Input: part model. Units: mm. Frame: model coordinates. Face numbers are marked on the shaded views. A direction names the side the tool comes from. Coordinates: 2 decimals unless noted, no trailing zeros. Order: outer loops, then holes, each group sorted by start corner. A loop starts at its lowest first (then second) coordinate and runs counter-clockwise, first axis right, second up. Notation, with made-up numbers: (7, 68.5) -> (40, 68.5) arc R20 cw to (40, 74.5) -> close; hole circle Ø3 at (-0.75, 83.5). An arc over 180 degrees is marked (long way). One line per item, written item: value. Start each with the question number.
from build123d import *

# Parameters (mm, degrees)
F0_R     = 70
F0_R_2   = 15
F1_DEPTH = 30
F3_DEPTH = 31


with BuildPart() as f1:
    # F0 (on Front) → F1 (new body)
    with BuildSketch(Plane.XZ):
        Circle(F0_R)
        Circle(F0_R_2, mode=Mode.SUBTRACT)
    extrude(amount=F1_DEPTH)

    # F2 (on face) → F3 (cut)
    with BuildSketch(Plane.XZ.offset(30)):
        with BuildLine():
            ThreePointArc((3.959342, 59.869221), (5.917735, 66.084931), (8.705645, 71.975425))
            ThreePointArc((8.705645, 71.975425), (0, 72.5), (-8.705645, 71.975425))
            ThreePointArc((-8.705645, 71.975425), (-5.917735, 66.084931), (-3.959342, 59.869221))
            ThreePointArc((-3.959342, 59.869221), (0, 60), (3.959342, 59.869221))
        make_face()
        with BuildLine():
            ThreePointArc((-11.670864, 58.85398), (-11.387945, 65.364764), (-10.219603, 71.776108))
            ThreePointArc((-10.219603, 71.776108), (-18.764381, 70.029622), (-27.037618, 67.269735))
            ThreePointArc((-27.037618, 67.269735), (-22.820132, 62.301519), (-19.319725, 56.804474))
            ThreePointArc((-19.319725, 56.804474), (-15.529143, 57.95555), (-11.670864, 58.85398))
        make_face()
        with BuildLine():
            ThreePointArc((-26.50572, 53.827937), (-27.917556, 60.190097), (-28.448402, 66.685369))
            ThreePointArc((-28.448402, 66.685369), (-36.25, 62.786842), (-43.527022, 57.979724))
            ThreePointArc((-43.527022, 57.979724), (-38.167375, 54.272361), (-33.363501, 49.868595))
            ThreePointArc((-33.363501, 49.868595), (-30, 51.961524), (-26.50572, 53.827937))
        make_face()
        with BuildLine():
            ThreePointArc((-39.534255, 45.13361), (-42.544632, 50.913574), (-44.73849, 57.050132))
            ThreePointArc((-44.73849, 57.050132), (-51.265242, 51.265242), (-57.050132, 44.73849))
            ThreePointArc((-57.050132, 44.73849), (-50.913574, 42.544632), (-45.13361, 39.534255))
            ThreePointArc((-45.13361, 39.534255), (-42.426407, 42.426407), (-39.534255, 45.13361))
        make_face()
        with BuildLine():
            ThreePointArc((-49.868595, 33.363501), (-54.272361, 38.167375), (-57.979724, 43.527022))
            ThreePointArc((-57.979724, 43.527022), (-62.786842, 36.25), (-66.685369, 28.448402))
            ThreePointArc((-66.685369, 28.448402), (-60.190097, 27.917556), (-53.827937, 26.50572))
            ThreePointArc((-53.827937, 26.50572), (-51.961524, 30), (-49.868595, 33.363501))
        make_face()
        with BuildLine():
            ThreePointArc((-56.804474, 19.319725), (-62.301519, 22.820132), (-67.269735, 27.037618))
            ThreePointArc((-67.269735, 27.037618), (-70.029622, 18.764381), (-71.776108, 10.219603))
            ThreePointArc((-71.776108, 10.219603), (-65.364764, 11.387945), (-58.85398, 11.670864))
            ThreePointArc((-58.85398, 11.670864), (-57.95555, 15.529143), (-56.804474, 19.319725))
        make_face()
        with BuildLine():
            ThreePointArc((-59.869221, 3.959342), (-66.084931, 5.917735), (-71.975425, 8.705645))
            ThreePointArc((-71.975425, 8.705645), (-72.5, 0), (-71.975425, -8.705645))
            ThreePointArc((-71.975425, -8.705645), (-66.084931, -5.917735), (-59.869221, -3.959342))
            ThreePointArc((-59.869221, -3.959342), (-60, 0), (-59.869221, 3.959342))
        make_face()
        with BuildLine():
            ThreePointArc((-58.85398, -11.670864), (-65.364764, -11.387945), (-71.776108, -10.219603))
            ThreePointArc((-71.776108, -10.219603), (-70.029622, -18.764381), (-67.269735, -27.037618))
            ThreePointArc((-67.269735, -27.037618), (-62.301519, -22.820132), (-56.804474, -19.319725))
            ThreePointArc((-56.804474, -19.319725), (-57.95555, -15.529143), (-58.85398, -11.670864))
        make_face()
        with BuildLine():
            ThreePointArc((-53.827937, -26.50572), (-60.190097, -27.917556), (-66.685369, -28.448402))
            ThreePointArc((-66.685369, -28.448402), (-62.786842, -36.25), (-57.979724, -43.527022))
            ThreePointArc((-57.979724, -43.527022), (-54.272361, -38.167375), (-49.868595, -33.363501))
            ThreePointArc((-49.868595, -33.363501), (-51.961524, -30), (-53.827937, -26.50572))
        make_face()
        with BuildLine():
            ThreePointArc((-45.13361, -39.534255), (-50.913574, -42.544632), (-57.050132, -44.73849))
            ThreePointArc((-57.050132, -44.73849), (-51.265242, -51.265242), (-44.73849, -57.050132))
            ThreePointArc((-44.73849, -57.050132), (-42.544632, -50.913574), (-39.534255, -45.13361))
            ThreePointArc((-39.534255, -45.13361), (-42.426407, -42.426407), (-45.13361, -39.534255))
        make_face()
        with BuildLine():
            ThreePointArc((-33.363501, -49.868595), (-38.167375, -54.272361), (-43.527022, -57.979724))
            ThreePointArc((-43.527022, -57.979724), (-36.25, -62.786842), (-28.448402, -66.685369))
            ThreePointArc((-28.448402, -66.685369), (-27.917556, -60.190097), (-26.50572, -53.827937))
            ThreePointArc((-26.50572, -53.827937), (-30, -51.961524), (-33.363501, -49.868595))
        make_face()
        with BuildLine():
            ThreePointArc((-19.319725, -56.804474), (-22.820132, -62.301519), (-27.037618, -67.269735))
            ThreePointArc((-27.037618, -67.269735), (-18.764381, -70.029622), (-10.219603, -71.776108))
            ThreePointArc((-10.219603, -71.776108), (-11.387945, -65.364764), (-11.670864, -58.85398))
            ThreePointArc((-11.670864, -58.85398), (-15.529143, -57.95555), (-19.319725, -56.804474))
        make_face()
        with BuildLine():
            ThreePointArc((-3.959342, -59.869221), (-5.917735, -66.084931), (-8.705645, -71.975425))
            ThreePointArc((-8.705645, -71.975425), (0, -72.5), (8.705645, -71.975425))
            ThreePointArc((8.705645, -71.975425), (5.917735, -66.084931), (3.959342, -59.869221))
            ThreePointArc((3.959342, -59.869221), (0, -60), (-3.959342, -59.869221))
        make_face()
        with BuildLine():
            ThreePointArc((11.670864, -58.85398), (11.387945, -65.364764), (10.219603, -71.776108))
            ThreePointArc((10.219603, -71.776108), (18.764381, -70.029622), (27.037618, -67.269735))
            ThreePointArc((27.037618, -67.269735), (22.820132, -62.301519), (19.319725, -56.804474))
            ThreePointArc((19.319725, -56.804474), (15.529143, -57.95555), (11.670864, -58.85398))
        make_face()
        with BuildLine():
            ThreePointArc((26.50572, -53.827937), (27.917556, -60.190097), (28.448402, -66.685369))
            ThreePointArc((28.448402, -66.685369), (36.25, -62.786842), (43.527022, -57.979724))
            ThreePointArc((43.527022, -57.979724), (38.167375, -54.272361), (33.363501, -49.868595))
            ThreePointArc((33.363501, -49.868595), (30, -51.961524), (26.50572, -53.827937))
        make_face()
        with BuildLine():
            ThreePointArc((39.534255, -45.13361), (42.544632, -50.913574), (44.73849, -57.050132))
            ThreePointArc((44.73849, -57.050132), (51.265242, -51.265242), (57.050132, -44.73849))
            ThreePointArc((57.050132, -44.73849), (50.913574, -42.544632), (45.13361, -39.534255))
            ThreePointArc((45.13361, -39.534255), (42.426407, -42.426407), (39.534255, -45.13361))
        make_face()
        with BuildLine():
            ThreePointArc((49.868595, -33.363501), (54.272361, -38.167375), (57.979724, -43.527022))
            ThreePointArc((57.979724, -43.527022), (62.786842, -36.25), (66.685369, -28.448402))
            ThreePointArc((66.685369, -28.448402), (60.190097, -27.917556), (53.827937, -26.50572))
            ThreePointArc((53.827937, -26.50572), (51.961524, -30), (49.868595, -33.363501))
        make_face()
        with BuildLine():
            ThreePointArc((56.804474, -19.319725), (62.301519, -22.820132), (67.269735, -27.037618))
            ThreePointArc((67.269735, -27.037618), (70.029622, -18.764381), (71.776108, -10.219603))
            ThreePointArc((71.776108, -10.219603), (65.364764, -11.387945), (58.85398, -11.670864))
            ThreePointArc((58.85398, -11.670864), (57.95555, -15.529143), (56.804474, -19.319725))
        make_face()
        with BuildLine():
            ThreePointArc((59.869221, -3.959342), (66.084931, -5.917735), (71.975425, -8.705645))
            ThreePointArc((71.975425, -8.705645), (72.5, 0), (71.975425, 8.705645))
            ThreePointArc((71.975425, 8.705645), (66.084931, 5.917735), (59.869221, 3.959342))
            ThreePointArc((59.869221, 3.959342), (60, 0), (59.869221, -3.959342))
        make_face()
        with BuildLine():
            ThreePointArc((58.85398, 11.670864), (65.364764, 11.387945), (71.776108, 10.219603))
            ThreePointArc((71.776108, 10.219603), (70.029622, 18.764381), (67.269735, 27.037618))
            ThreePointArc((67.269735, 27.037618), (62.301519, 22.820132), (56.804474, 19.319725))
            ThreePointArc((56.804474, 19.319725), (57.95555, 15.529143), (58.85398, 11.670864))
        make_face()
        with BuildLine():
            ThreePointArc((53.827937, 26.50572), (60.190097, 27.917556), (66.685369, 28.448402))
            ThreePointArc((66.685369, 28.448402), (62.786842, 36.25), (57.979724, 43.527022))
            ThreePointArc((57.979724, 43.527022), (54.272361, 38.167375), (49.868595, 33.363501))
            ThreePointArc((49.868595, 33.363501), (51.961524, 30), (53.827937, 26.50572))
        make_face()
        with BuildLine():
            ThreePointArc((45.13361, 39.534255), (50.913574, 42.544632), (57.050132, 44.73849))
            ThreePointArc((57.050132, 44.73849), (51.265242, 51.265242), (44.73849, 57.050132))
            ThreePointArc((44.73849, 57.050132), (42.544632, 50.913574), (39.534255, 45.13361))
            ThreePointArc((39.534255, 45.13361), (42.426407, 42.426407), (45.13361, 39.534255))
        make_face()
        with BuildLine():
            ThreePointArc((33.363501, 49.868595), (38.167375, 54.272361), (43.527022, 57.979724))
            ThreePointArc((43.527022, 57.979724), (36.25, 62.786842), (28.448402, 66.685369))
            ThreePointArc((28.448402, 66.685369), (27.917556, 60.190097), (26.50572, 53.827937))
            ThreePointArc((26.50572, 53.827937), (30, 51.961524), (33.363501, 49.868595))
        make_face()
        with BuildLine():
            ThreePointArc((19.319725, 56.804474), (22.820132, 62.301519), (27.037618, 67.269735))
            ThreePointArc((27.037618, 67.269735), (18.764381, 70.029622), (10.219603, 71.776108))
            ThreePointArc((10.219603, 71.776108), (11.387945, 65.364764), (11.670864, 58.85398))
            ThreePointArc((11.670864, 58.85398), (15.529143, 57.95555), (19.319725, 56.804474))
        make_face()
    extrude(amount=-F3_DEPTH, mode=Mode.SUBTRACT)


solid = f1.part
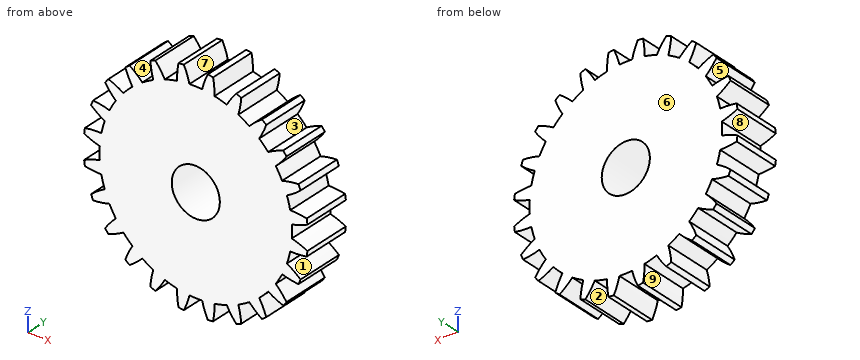
1) Pin query (flat end, axial travel): pin 1 Ø6 at (y, z) = (-19, -34.5) entering from +X; pin 2 Ø1 at (y, z) = (-15, 27.5) entering from -X; pin 3 Ø1.5 at (x, y) = (32.5, -14) entering from -Z. Return the tip coordinate at first contact, or that it passes through.
2) Mould query, pull axis X, two halves, no side actions, for the marked faces 6, 7, 8 and 9. Classes: +X half, -X half, draft (parallel to the pull), parting line (faces both ways), or undercut.
3) Section query D-D, the plane z = 35.5. Return the cut outline in (x, y).
4) Ray query, line 1 along Z through (x, y) = (0, -11); line 2 along X through (y, z) = (-21.5, 51.5); line 3 along Z through (x, y) = (53, -13.5). Return the intervals inside material, ascending. Write a range as from..to.
5) Section query C-C, the plane x = 21. Return the cut outline in (y, z).
6) Access query for the marked faces 1, 2, 3, 4 and 5. Directions: +Z, -Z, +X, -X, +Y, -Y. A direction counts if a zero-diameter tool reaches every point of the face in a straight line with its end or side. Return the directions, or none.
7) Section query B-B, the plane z = 0. Return the cut outline in (x, y).
8) Section query A-A, the plane x = 0. Return the cut outline in (y, z), plus the area to 3 significant figures.
Entries:
1. pin 1: stops at x = 53.73
1. pin 2: stops at x = -64.58
1. pin 3: stops at z = -50.91
2. face 6: draft
2. face 7: undercut
2. face 8: -X half
2. face 9: undercut
3. outline: (-51.98, -30) -> (51.98, -30) -> (51.98, 0) -> (-51.98, 0) -> close
4. line 1: z = -60..-15, 15..60
4. line 2: x = -42.8..-34.99, -30.79..30.79, 34.99..42.8
4. line 3: z = -43.4..-36.64, -28.12..28.12, 36.64..43.4
5. outline: (-30, -59.65) -> (0, -59.65) -> (0, 59.65) -> (-30, 59.65) -> close
6. face 1: +X, +Y, -Y
6. face 2: -Z, +Y, -Y
6. face 3: +Y, -Y
6. face 4: +Z, +Y, -Y
6. face 5: -X, +Y, -Y
7. outline: (-60, -30) -> (-15, -30) -> (-15, 0) -> (-60, 0) -> close; (15, -30) -> (60, -30) -> (60, 0) -> (15, 0) -> close
8. outline: (-30, -60) -> (0, -60) -> (0, -15) -> (-30, -15) -> close; (-30, 15) -> (0, 15) -> (0, 60) -> (-30, 60) -> close
8. area: 2,700 mm2
